Solid Edge part; units mm, degrees
sketch "Sketch1" plane through (0, 0, 0) normal (0, 0, 1) x (1, 0, 0)
  circle A0 centre (45.72, -45.72) radius 1.6
  line L0 (-49.53, 44.53) -> (-49.53, -68.72)
  arc A1 (-49.53, -68.72) -> (-46.03, -72.22) centre (-46.03, -68.72) ccw
  line L1 (-46.03, -72.22) -> (46.03, -72.22)
  arc A2 (49.53, -68.72) -> (46.03, -72.22) centre (46.03, -68.72) cw
  line L2 (49.53, 44.53) -> (49.53, -68.72)
  arc A3 (44.53, 49.53) -> (49.53, 44.53) centre (44.53, 44.53) cw
  line L3 (44.53, 49.53) -> (-44.53, 49.53)
  arc A4 (-44.53, 49.53) -> (-49.53, 44.53) centre (-44.53, 44.53) ccw
  circle A5 centre (45.72, 45.72) radius 1.6
  circle A6 centre (-45.72, -45.72) radius 1.6
  circle A7 centre (-45.72, 45.72) radius 1.6
  circle A8 centre (45.72, -68.41) radius 1.6
  circle A9 centre (-45.72, -68.41) radius 1.6
  circle A10 centre (0, -12.5) radius 2.5
  circle A11 centre (20, 0) radius 2.5
  circle A12 centre (0, 20) radius 2.5
  circle A13 centre (0, 0) radius 2.5
  circle A14 centre (-20, 0) radius 2.5
  circle A15 centre (0, 12.5) radius 2.5
  circle A16 centre (12.5, 0) radius 2.5
  circle A17 centre (0, -20) radius 2.5
  circle A18 centre (-12.5, 0) radius 2.5
extrude "Protrusion1" add sketch "Sketch1" along normal blind 3
properties material "Acrylic, high impact grade"
The listing builds one solid part. Answer for the finished solid, in the listing's coordinates (mm). Give positions to 0.01 mm unless a question says otherwise; leave off trailing zeros. Write each loop counter-clockwise with the first axis right and the second up, starting at its lowest first coordinate (ties: lowest second). Pieces come first, ordered by that corner, then holes.
1) Section C-C (z = 1.8) is taken. Count the separate pieces of the cut face and the enclosed holes in it, and give its area (3 significant figures).
2) For a pull along X with two mould halves and no side action, classify faces 1 (the face through (10, -10, 3)), 2 (the face through (48.5, -71.2, 1.5)), 3 (the face through (10, 0, 1)) as pulls with the +X half, pulls with the -X half, needs draft (parallel to the pull), parting line crosses it, or undercut.
3) Section D-D (y = 0) is taken. Write down the section's boundary in (x, z), and give its area (3 significant figures).
4) Section B-B (x = -12.5) is taken. Write down the section's boundary in (y, z).
5) Section A-A (y = 12.5) is taken. Write down the section's boundary in (x, z).
6) Find the intervals of material crossed by L1, parallel to X at y = -68.41, z = 2.25; L2, parallel to Y at x = 1.5, z = 0.3; L3, parallel to X at y = -1, z = 1.35, in increasing order.
Response:
1. separate pieces: 1
1. enclosed holes: 15
1. area: 11,800 mm2
2. face 1: needs draft
2. face 2: pulls with the +X half
2. face 3: undercut
3. outline: (-49.53, 0) - (-22.5, 0) - (-22.5, 3) - (-49.53, 3) - close; (-17.5, 0) - (-15, 0) - (-15, 3) - (-17.5, 3) - close; (-10, 0) - (-2.5, 0) - (-2.5, 3) - (-10, 3) - close; (2.5, 0) - (10, 0) - (10, 3) - (2.5, 3) - close; (15, 0) - (17.5, 0) - (17.5, 3) - (15, 3) - close; (22.5, 0) - (49.53, 0) - (49.53, 3) - (22.5, 3) - close
3. area: 222 mm2
4. outline: (-72.22, 0) - (-2.5, 0) - (-2.5, 3) - (-72.22, 3) - close; (2.5, 0) - (49.53, 0) - (49.53, 3) - (2.5, 3) - close
5. outline: (-49.53, 0) - (-2.5, 0) - (-2.5, 3) - (-49.53, 3) - close; (2.5, 0) - (49.53, 0) - (49.53, 3) - (2.5, 3) - close
6. L1: x = -49.53 to -47.32, -44.12 to 44.12, 47.32 to 49.53
6. L2: y = -72.22 to -22, -18 to -14.5, -10.5 to -2, 2 to 10.5, 14.5 to 18, 22 to 49.53
6. L3: x = -49.53 to -22.29, -17.71 to -14.79, -10.21 to -2.29, 2.29 to 10.21, 14.79 to 17.71, 22.29 to 49.53
